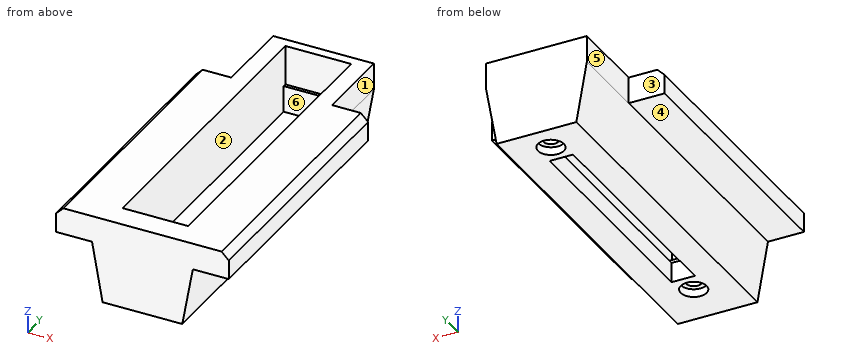
```python
from build123d import *

# Parameters (mm, degrees)
EXTRUDE_1_DEPTH     = 40
EXTRUDE_2_DEPTH     = 12
CHAMFER_1_SIZE      = 1.1
SKETCH_3_W          = 9.9
SKETCH_3_H          = 45.3
CUT_EXTRUDE_1_DEPTH = 10
SKETCH_4_W          = 3.5
SKETCH_4_H          = 35
CUT_EXTRUDE_2_DEPTH = 55.525223521
SKETCH_5_W          = 9.9
SKETCH_5_H          = 0.5
SKETCH_5_H_2        = 1
CUT_EXTRUDE_3_DEPTH = 6
SKETCH_6_R          = 1.15
CUT_EXTRUDE_4_DEPTH = 55.525223521
SKETCH_7_R          = 1.95
CUT_EXTRUDE_5_DEPTH = 1.2


with BuildPart() as part:
    # 草图1 → 凸台-拉伸1 (new body)
    with BuildSketch(Plane(origin=(0, 0, 0), x_dir=(1, 0, 0), z_dir=(0, 1, 0))):
        Polygon((-13, 0), (13, 0), (13, 4), (7.586942826, 4), (6, 13), (-6, 13), (-7.586942826, 4), (-13, 4), align=None)
    extrude(amount=EXTRUDE_1_DEPTH)

    # 草图2 → 凸台-拉伸2 (add)
    with BuildSketch(Plane(origin=(0, 40, 0), x_dir=(1, 0, 0), z_dir=(0, 1, 0))):
        Polygon((7.586942826, 4), (6, 13), (-6, 13), (-7.586942826, 4), (-7.586942826, 0), (7.586942826, 0), align=None)
    extrude(amount=EXTRUDE_2_DEPTH)

    # 倒角1
    chamfer_1_edges = [part.edges().sort_by_distance(p)[0] for p in [
        (13, 20, 0),
        (-13, 20, 0),
    ]]
    chamfer(chamfer_1_edges, length=CHAMFER_1_SIZE)

    # 草图3 → 切除-拉伸1 (cut)
    with BuildSketch(Plane.XY):
        with Locations((0, 27.35)):
            Rectangle(SKETCH_3_W, SKETCH_3_H)
    extrude(amount=-CUT_EXTRUDE_1_DEPTH, mode=Mode.SUBTRACT)

    # 草图4 → 切除-拉伸2 (cut, through all)
    with BuildSketch(Plane.XY.offset(-10)):
        with Locations((0, 27.35)):
            Rectangle(SKETCH_4_W, SKETCH_4_H)
    extrude(amount=-CUT_EXTRUDE_2_DEPTH, mode=Mode.SUBTRACT)

    # 草图5 → 切除-拉伸3 (cut)
    with BuildSketch(Plane.XY):
        with Locations((0, 50.25)):
            Rectangle(SKETCH_5_W, SKETCH_5_H)
        with Locations((0, 4.2)):
            Rectangle(SKETCH_5_W, SKETCH_5_H_2)
    extrude(amount=-CUT_EXTRUDE_3_DEPTH, mode=Mode.SUBTRACT)

    # 草图6 → 切除-拉伸4 (cut, through all)
    with BuildSketch(Plane.XY.offset(-10)):
        with Locations((0, 47.85)):
            Circle(SKETCH_6_R)
        with Locations(Location((0, 6.85, 0), (0, 0, 180))):
            Circle(SKETCH_6_R)
    extrude(amount=-CUT_EXTRUDE_4_DEPTH, mode=Mode.SUBTRACT)

    # 草图7 → 切除-拉伸5 (cut)
    with BuildSketch(Plane(origin=(0, 0, -13), x_dir=(-1, 0, 0), z_dir=(0, 0, -1))):
        with Locations((0, 47.85)):
            Circle(SKETCH_7_R)
        with Locations((0, 6.85)):
            Circle(SKETCH_7_R)
    extrude(amount=-CUT_EXTRUDE_5_DEPTH, mode=Mode.SUBTRACT)


solid = part.part
```
The listing builds one solid part. Answer for the finished solid, in the listing's coordinates (mm). Face numbers are marked on the shaded views. A direction names the side the tool comes from. Give positions to 0.01 mm unless a question says otherwise; leave off trailing zeros. Order: outer loops, then holes, each group sorted by start corner. A loop starts at its lowest first (then second) coordinate and runs counter-clockwise, first axis right, second up. Notation, with made-up numbers: (-40, -32.5) -> (-34, -32.5) arc R6 ccw to (-34, -25.5) -> close; hole circle Ø7 at (40.5, -6.75). An arc over 180 degrees is marked (long way). Answer as a JSON object with one key per item and string values. Group by question number.
Item 1: The part is cut by section C-C on z = -8.25. Write down the section's boundary in (x, y).
Item 2: Determine the mould class of the marked faces 1, 2 and 3 for opening direction X: pulls with the +X half, pulls with the -X half, needs draft (parallel to the pull), parting line crosses it, or undercut.
Item 3: A tool of negligible diameter and unlimited length cuts with its end or side. For the marked faces 4, 5 and 6, from which of +Z, -Z, +X, -X, +Y, -Y can it reach the whole face along a straight path? Write none if from no direction.
Item 4: The part is cut by section D-D on y = 31. Write down the section's boundary in (x, z).
Item 5: The part is cut by section A-A on y = 40.5. Write down the section's boundary in (x, z).
Item 6: Flat-ended cylindrical pins translate along their axes: pin 1 (3 mm diameter, centred on y = 49, z = -1, fed in from +X); pin 2 (2.5 mm diameter, centred on x = 0, y = 6.85, fed in from -Z); pin 3 (1.5 mm diameter, centred on y = 29, z = -10.5, fed in from +X). Find the tip coordinate at first contact, or state that the pin passes through.
Item 7: Consider L1, parallel to Y at x = 0, z = -12.1; L2, parallel to Y at x = 0, z = -10.5; L3, parallel to Y at x = 2.75, z = -2.5. Determine where each line is inside the solid, lowest interval first. Write a range as from..to.
Item 8: The part is cut by section B-B on x = 0. Give the number of separate pieces and of enclosed holes in the cut face, and give its area (3 significant figures).
Result set:
{
 "1": {"outline": "(-6.84, 0) -> (6.84, 0) -> (6.84, 52) -> (-6.84, 52) -> close; hole (-4.95, 4.7) -> (4.95, 4.7) -> (4.95, 50) -> (-4.95, 50) -> close"},
 "2": {"face 1": "pulls with the +X half", "face 2": "undercut", "face 3": "needs draft"},
 "3": {"face 4": "-Z, -X, +Y, -Y", "face 5": "+Z, -Z, -X, +Y", "face 6": "+Z"},
 "4": {"outline": "(-13, -4) -> (-7.59, -4) -> (-6, -13) -> (-1.75, -13) -> (-1.75, -10) -> (-4.95, -10) -> (-4.95, 0) -> (-11.9, 0) -> (-13, -1.1) -> close; (1.75, -13) -> (6, -13) -> (7.59, -4) -> (13, -4) -> (13, -1.1) -> (11.9, 0) -> (4.95, 0) -> (4.95, -10) -> (1.75, -10) -> close"},
 "5": {"outline": "(-7.59, -4) -> (-6, -13) -> (-1.75, -13) -> (-1.75, -10) -> (-4.95, -10) -> (-4.95, 0) -> (-7.59, 0) -> close; (1.75, -13) -> (6, -13) -> (7.59, -4) -> (7.59, 0) -> (4.95, 0) -> (4.95, -10) -> (1.75, -10) -> close"},
 "6": {"pin 1": "x = 7.59", "pin 2": "z = -11.8", "pin 3": "x = 6.57"},
 "7": {"L1": "0..4.9, 8.8..9.85, 44.85..45.9, 49.8..52", "L2": "0..5.7, 8..9.85, 44.85..46.7, 49..52", "L3": "0..3.7, 50.5..52"},
 "8": {"separate pieces": "4", "enclosed holes": "0", "area": "91.4 mm²"}
}
